from build123d import *

# Parameters (mm, degrees)
SKETCH1_W               = 17
SKETCH1_H               = 14
SKETCH1_W_2             = 6
SKETCH1_H_2             = 6
BOSS_EXTRUDE1_DEPTH     = 3.2
CUT_EXTRUDE1_DEPTH      = 12.466908912
CUT_EXTRUDE1_DEPTH_BACK = 12.466908912
SKETCH2_R               = 2


with BuildPart() as part:
    # Sketch1 → Boss-Extrude1 (new, symmetric)
    with BuildSketch(Plane(origin=(0, 0, 0), x_dir=(1, 0, 0), z_dir=(0, 1, 0))):
        Rectangle(SKETCH1_W, SKETCH1_H)
        Rectangle(SKETCH1_W_2, SKETCH1_H_2, mode=Mode.SUBTRACT)
    extrude(amount=BOSS_EXTRUDE1_DEPTH, both=True)

    # Sketch2 → Cut-Extrude1 (cut, two sides: drawn at the far end of the back side and taken through both)
    with BuildSketch(Plane(origin=(0, 0, 0), x_dir=(0, 0, -1), z_dir=(1, 0, 0)).offset(-CUT_EXTRUDE1_DEPTH_BACK)):
        Circle(SKETCH2_R)
    extrude(amount=CUT_EXTRUDE1_DEPTH + CUT_EXTRUDE1_DEPTH_BACK, mode=Mode.SUBTRACT)


solid = part.part
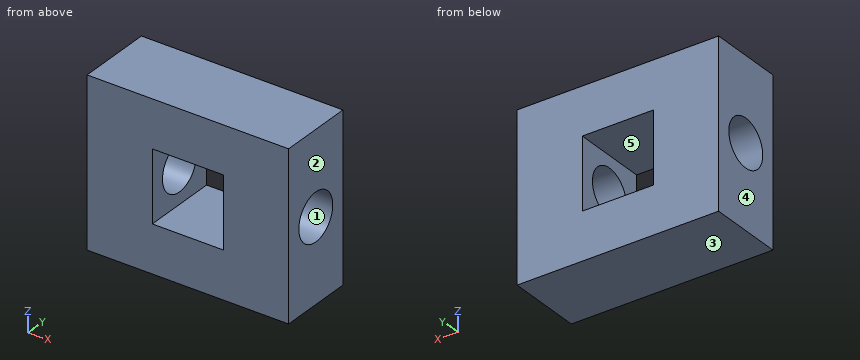
For this review, take the finished solid that the model builds, in its own axes (mm). Face numbers are marked on the shaded views. A direction names the side the tool comes from. Coordinates: 2 decimals unless noted, no trailing zeros. Order: outer loops, then holes, each group sorted by start corner. A loop starts at its lowest first (then second) coordinate and runs counter-clockwise, first axis right, second up. Notation, with made-up numbers: (27.5, -28.75) - (49.5, -28.75) arc R27 cw to (49.5, -5.75) - close; hole circle Ø2 at (-32, -29). An arc over 180 degrees is marked (long way). Answer as CSV lines item,"result". Start each with the question number.
1) Add section B-B (y = 0). State the section outline as (x, z) points.
2) Draft analysis for pull direction Z (two halves, no side actions). For the marked faces 1, 2 and 3, state which applies: +Z half, -Z half, draft (parallel to the pull), parting line (faces both ways), or undercut.
3) Add section D-D (y = 2.75). State the section outline as (x, z) points.
4) Machinability: for the marked faces 4 and 5, which of the approach directions +Z, -Z, +X, -X, +Y, -Y give a long, thin tool a straight path to every point of the face, cutting with its end or side? Answer none if there is none.
5) Add section A-A (x = -0.75). State the section outline as (y, z) points.
6) Add section C-C (z = 0). State the section outline as (x, y) points, then the cut area to 3 significant figures.
7) Insertion check: P1, Ø3, axis at y = 0, z = 0, coming from the +X side. The pin has a flat end and moves straight along its axis. Give the tip position at first contact, or say it passes through.
8) To check wall thickness, follow line 1 along Z through (x, y) = (-2.75, -1); line 2 along Y through (x, z) = (4.35, 0); line 3 along X through (y, z) = (2.25, 1). State the ranges of each line that lie inside material, in increasing order. Write a range as [from, to].
Result:
1,outline,"(-8.5, -7) - (8.5, -7) - (8.5, -2) - (3, -2) - (3, -3) - (-3, -3) - (-3, -2) - (-8.5, -2) - close; (-8.5, 2) - (-3, 2) - (-3, 3) - (3, 3) - (3, 2) - (8.5, 2) - (8.5, 7) - (-8.5, 7) - close"
2,face 1,"undercut"
2,face 2,"draft"
2,face 3,"-Z half"
3,outline,"(-8.5, -7) - (8.5, -7) - (8.5, 7) - (-8.5, 7) - close; hole (-3, -3) - (3, -3) - (3, 3) - (-3, 3) - close"
4,face 4,"+Z, -Z, -X, +Y, -Y"
4,face 5,"+Y, -Y"
5,outline,"(-3.2, -7) - (3.2, -7) - (3.2, -3) - (-3.2, -3) - close; (-3.2, 3) - (3.2, 3) - (3.2, 7) - (-3.2, 7) - close"
6,outline,"(-8.5, -3.2) - (-3, -3.2) - (-3, -2) - (-8.5, -2) - close; (-8.5, 2) - (-3, 2) - (-3, 3.2) - (-8.5, 3.2) - close; (3, -3.2) - (8.5, -3.2) - (8.5, -2) - (3, -2) - close; (3, 2) - (8.5, 2) - (8.5, 3.2) - (3, 3.2) - close"
6,area,"26.4 mm^2"
7,P1,"through"
8,line 1,"[-7, -3], [3, 7]"
8,line 2,"[-3.2, -2], [2, 3.2]"
8,line 3,"[-8.5, -3], [3, 8.5]"
